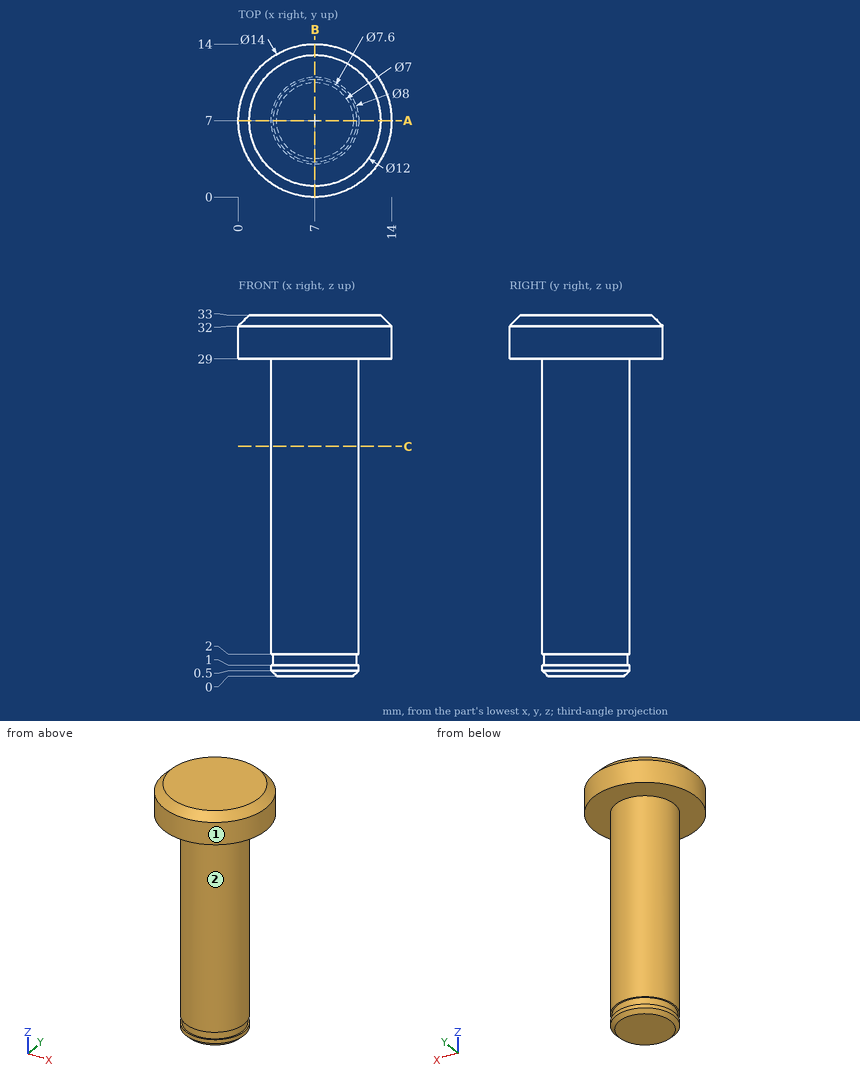
Print and shaded views of the part. All mm, measured from the part's lowest x, y and z. A direction names the side the tool comes from. Coordinates: 2 decimals unless noted, no trailing zeros. Write each loop counter-clockwise with the first axis right and the second up, starting at its lowest first coordinate (ties: lowest second). Pieces come first, ordered by that corner, then holes. Notation, with made-up numbers: (45, -29) - (82, -29) arc R19 cw to (82, -15) - close; hole circle Ø5 at (87, 83.25). An arc over 180 degrees is marked (long way). One line per question, with ' | ' between items. Start each with the question number.
Q1. Drill centre lines: line 1 (Z direction, x = 2, y = 7); line 2 (X direction, y = 5.75, z = 3); line 3 (X direction, y = 9.25, z = 6). Where is each one in solid material? Low to high. Write a range as [from, to].
Q2. Cut at A-A, the plane y = 7. List the corners of the cut face in (x, z).
Q3. Pin check, flat tips, straight feed: pin 1 (4 mm diameter, centred on y = 9, z = 18.5, fed in from -X); pin 2 (1.5 mm diameter, centred on x = 10, z = 17.5, fed in from -Y); pin 3 (5 mm diameter, centred on y = 6, z = 4.5, fed in from +X). Stop position of each tip, or through.
Q4. Cut at C-C, the plane z = 21. List the corners of the cut face in (x, y).
Q5. 3-axis set-ups, long thin cutter, end or side, ignore diameter. For the marked faces 1 and 2: which of +Z, -Z, +X, -X, +Y, -Y reach the whole face in a straight line?
Answer below:
1) line 1: [29, 33] | line 2: [3.2, 10.8] | line 3: [3.69, 10.31]
2) outline: (0, 29) - (3, 29) - (3, 2) - (3.2, 2) - (3.2, 1) - (3, 1) - (3, 0.5) - (3.5, 0) - (10.5, 0) - (11, 0.5) - (11, 1) - (10.8, 1) - (10.8, 2) - (11, 2) - (11, 29) - (14, 29) - (14, 32) - (13, 33) - (1, 33) - (0, 32) - close
3) pin 1: x = 3 | pin 2: y = 3.69 | pin 3: x = 11
4) outline: circle Ø8 at (7, 7)
5) face 1: +Z, -Z | face 2: -Z
